Geometry check sheet. Reference: drawing and pictorial views, mm from the part's lowest x, y, z. A direction names the side the tool comes from. Coordinates: 2 decimals unless noted, no trailing zeros. Write each loop counter-clockwise with the first axis right and the second up, starting at its lowest first coordinate (ties: lowest second). Pieces come first, ordered by that corner, then holes. Notation, with made-up numbers: (2.25, -30) - (25.25, -30) arc R16 ccw to (25.25, -14) - close; hole circle Ø1 at (-25.75, 78.25). An arc over 180 degrees is marked (long way). Use one line per item in the form item = value. Start each with the question number.
(1) Sectioned sample at D-D (y = 10). Record the cut outline in (x, z), and give its area (3 significant figures).
(2) Sectioned sample at B-B (z = 4). Record the cut outline in (x, y) (1 decimal).
(3) Sectioned sample at A-A (x = 7). Record the cut outline in (y, z).
(4) Sectioned sample at C-C (x = 1.75). Record the cut outline in (y, z), and give its area (3 significant figures).
(5) Gauge pin test, flat ends, axial feed: pin 1 Ø5 at (x, z) = (9, 5) entering from -Y; pin 2 Ø3 at (y, z) = (7, 4) entering from -X; pin 3 Ø3 at (y, z) = (16.5, 8.5) entering from -X. Record the tip position at first contact, or that the pin passes through.
(6) Tool access check on the marked faces 1 and 2. Record the directions out of +Z, -Z, +X, -X, +Y, -Y that give a thin tool (end or side, any length) a straight path to the whole face; none if there is none.
(7) Material ranges on line 1 (Z direction, x = 5, y = 6); line 2 (Y direction, x = 9.5, z = 4.5); line 3 (Y direction, x = 4.5, z = 8.25), recorded low to high. Write a range as [from, to].
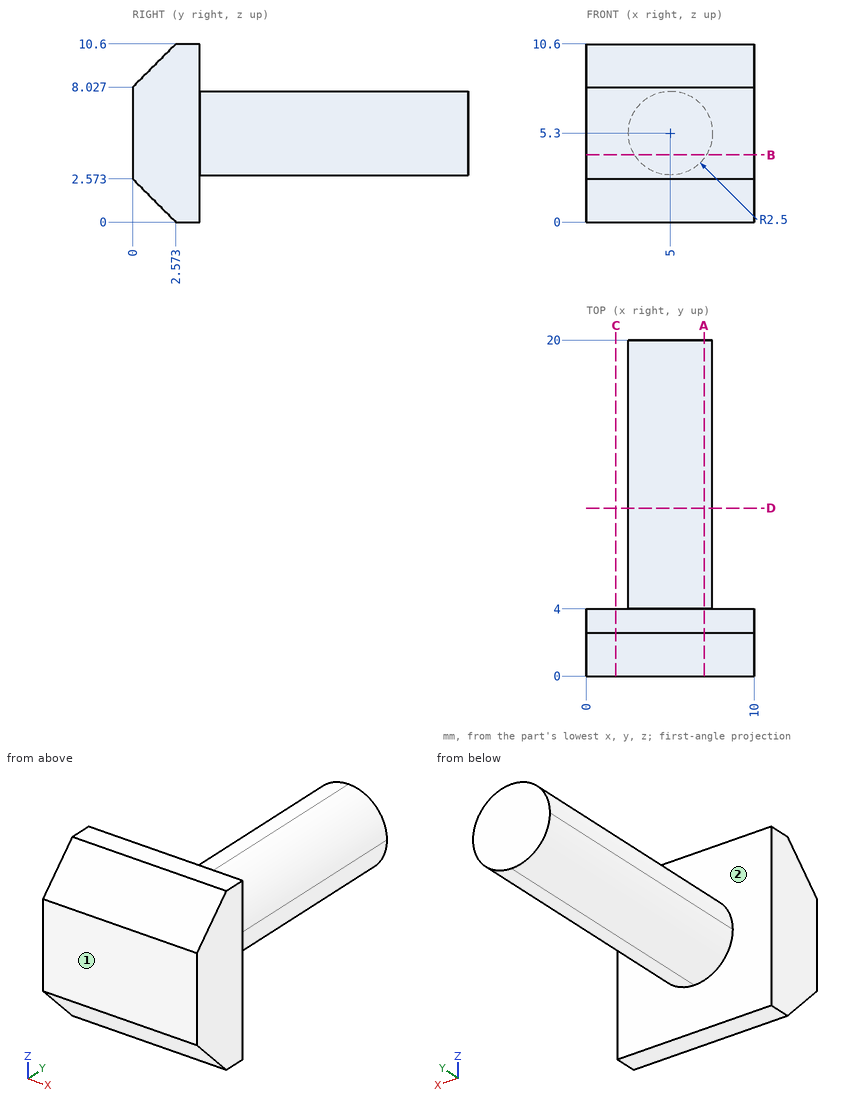
Answers below:
q1.outline = circle Ø5 at (5, 5.3)
q1.area = 19.6 mm2
q2.outline = (0, 0) - (10, 0) - (10, 4) - (7.1, 4) - (7.1, 20) - (2.9, 20) - (2.9, 4) - (0, 4) - close
q3.outline = (0, 2.57) - (2.57, 0) - (4, 0) - (4, 3.8) - (20, 3.8) - (20, 6.8) - (4, 6.8) - (4, 10.6) - (2.57, 10.6) - (0, 8.03) - close
q4.outline = (0, 2.57) - (2.57, 0) - (4, 0) - (4, 10.6) - (2.57, 10.6) - (0, 8.03) - close
q4.area = 35.8 mm2
q5.pin_1 = 0
q5.pin_2 = 2.5
q5.pin_3 = 3.17
q6.face_1 = +Z, -Z, +X, -X, -Y
q6.face_2 = +Y
q7.line_1 = [2.8, 7.8]
q7.line_2 = [0, 4]
q7.line_3 = [0.22, 4]
